Geometry check sheet. Reference: the model listing, model coordinates, mm. A direction names the side the tool comes from. Coordinates: 2 decimals unless noted, no trailing zeros. Write each loop counter-clockwise with the first axis right and the second up, starting at its lowest first coordinate (ties: lowest second). Pieces come first, ordered by that corner, then holes. Notation, with made-up numbers: M 81,76 L 115,76 A22 ccw 115,106 Z; hole C 10.5,3.25 d6. An arc over 180 degrees is marked long. Answer as a JSON object with one key per item and string values. Group by question number.
Autodesk Inventor part; units mm, degrees
ref_plane "YZ Plane" through (0, 0, 0) normal (1, 0, 0) x (0, 1, 0)
ref_plane "XZ Plane" through (0, 0, 0) normal (0, 1, 0) x (-1, 0, 0)
ref_plane "XY Plane" through (0, 0, 0) normal (0, 0, 1) x (1, 0, 0)
sketch "Skizze1" plane through (0, 0, 0) normal (0, 0, 1) x (1, 0, 0)
  line L0 (-15, 0) -> (15, 0)
  line L1 (-5.5, 5.1) -> (-2.75, 6.7)
  line L2 (-2.75, 6.7) -> (0, 5.1)
  line L3 (0, 5.1) -> (2.75, 6.7)
  line L4 (2.75, 6.7) -> (5.5, 5.1)
  line L5 (-5.5, 5.1) -> (5.5, 5.1) construction
  line L6 (-2.75, 6.7) -> (2.75, 6.7) construction
  line L7 (0, 5.1) -> (5.5, 5.1) construction
  line L8 (5.5, 6.0256) -> (2.75, 7.6256)
  line L9 (2.75, 7.6256) -> (0, 6.0256)
  line L10 (0, 6.0256) -> (-2.75, 7.6256)
  line L11 (-2.75, 7.6256) -> (-5.5, 6.0256)
  line L12 (-5.5, 5.1) -> (-7.9, 5.1)
  line L13 (-7.9, 5.1) -> (-7.9, 3)
  line L14 (-7.9, 3) -> (-9.5, 3)
  line L15 (-9.5, 3) -> (-9.5, 7.1)
  line L16 (-9.5, 7.1) -> (-5.5, 7.1)
  line L17 (-5.5, 7.1) -> (-5.5, 6.0256)
  line L18 (5.5, 5.1) -> (5.5, 6.0256)
  line L19 (4.5639, 6.5702) -> (5.5, 7.5)
  line L20 (5.5, 7.5) -> (5.5, 6.0256)
  line L21 (5.5, 7.5) -> (6.3, 7.5)
  line L22 (6.3, 7.5) -> (6.3, 5.1)
  line L23 (6.3, 5.1) -> (5.5, 5.1)
  line L24 (5.5, 5.1) -> (5.5, 7.5)
  line L25 (-0.75, 5.1) -> (0.75, 5.1)
  line L26 (0.75, 5.1) -> (0.75, 5.5364)
  line L27 (0.75, 5.5364) -> (-0.75, 5.5364)
  line L28 (-0.75, 5.5364) -> (-0.75, 5.1)
  point P0 (0, 0)
  point P1 (0, 0)
  point P2 (0, 6.7)
  point P3 (2.75, 5.1)
  point P4 (0, 5.5364)
  point P5 (-0.75, 5.5364)
  dimension "d37" = 0.8
  dimension "d38" = 6
  dimension "d39" = 10.2
  dimension "d40" = 2
  dimension "d41" = 1.6
  dimension "d42" = 11
  dimension "d43" = 4
  dimension "d44" = 1.6
  dimension "d45" = 30
  dimension "d46" = 75
  dimension "d47" = 15
  dimension "d49" = 0.8
  dimension "d50" = 1.5
revolve "Umdrehung2" add sketch "Skizze1" angle 360 about axis through (-15, 0, 0) along (1, 0, 0)
chamfer "Fase3" distance 0.5 angle 45 3 edges at (-2.75, -7.6256, 0) (2.75, -7.6256, 0) (0, -6.0256, 0)
properties part number "Daemper_TPU_Z2" material "Thermoplastisches Harz"
1) Section check A-A (x = -2). Record the cut outline in (y, z).
2) Set-up check for faces 1 (the flat face through (-5.5, -2, -6)), 2 (the flat face through (-9.5, 1, -3)), 3 (the cylindrical face through (-6.7, 2.4, 4.5)): record each of +Z, -Z, +X, -X, +Y, -Y from which the full face is reachable in a straight line by a thin tool's end or side.
3) Section check B-B (x = -4). Record the cut outline in (y, z).
4) Material ranges on probe 1 along X at (y, z) = (3.5, -4.5); probe 2 along X at (y, z) = (-0.25, 5.5); probe 3 along Z at (x, y) = (-0.2, 0), recorded low to high. Write a range as [from, to].
5) Go/stop test with flat-tipped pins: pin 1 Ø8 at (x, y) = (-5, -5.5) entering from +Z; pin 2 Ø3 at (y, z) = (-3.5, -0.5) entering from +X; pin 3 Ø2 at (x, y) = (-2.5, -1) entering from +Z. Record where each tip stops, or that it passes through.
6) Draft check along Z on faces 4 (the cylindrical face through (-7.47, -0.92, 7.04)), 5 (the flat face through (6.3, 2, -5)), 6 (the cylindrical face through (0, 2.4, -4.5)). Enter one of: +Z half, -Z half, draft (parallel to the pull), parting line (faces both ways), or undercut.
Entries:
{
 "1": {"outline": "C 0,0 d14.38; hole C 0,0 d12.53"},
 "2": {"face 1": "none", "face 2": "+Z, -Z, -X, +Y, -Y", "face 3": "+X"},
 "3": {"outline": "C 0,0 d13.8; hole C 0,0 d11.95"},
 "4": {"probe 1": "[-9.5, -4.47], [-1.03, 1.03], [4.47, 6.3]", "probe 2": "[-9.5, -4.8], [-0.75, 0.75], [4.8, 6.3]", "probe 3": "[-6.28, -5.1], [5.1, 6.28]"},
 "5": {"pin 1": "z = 7.12", "pin 2": "x = -7.9", "pin 3": "z = 7.37"},
 "6": {"face 4": "parting line", "face 5": "draft", "face 6": "undercut"}
}
